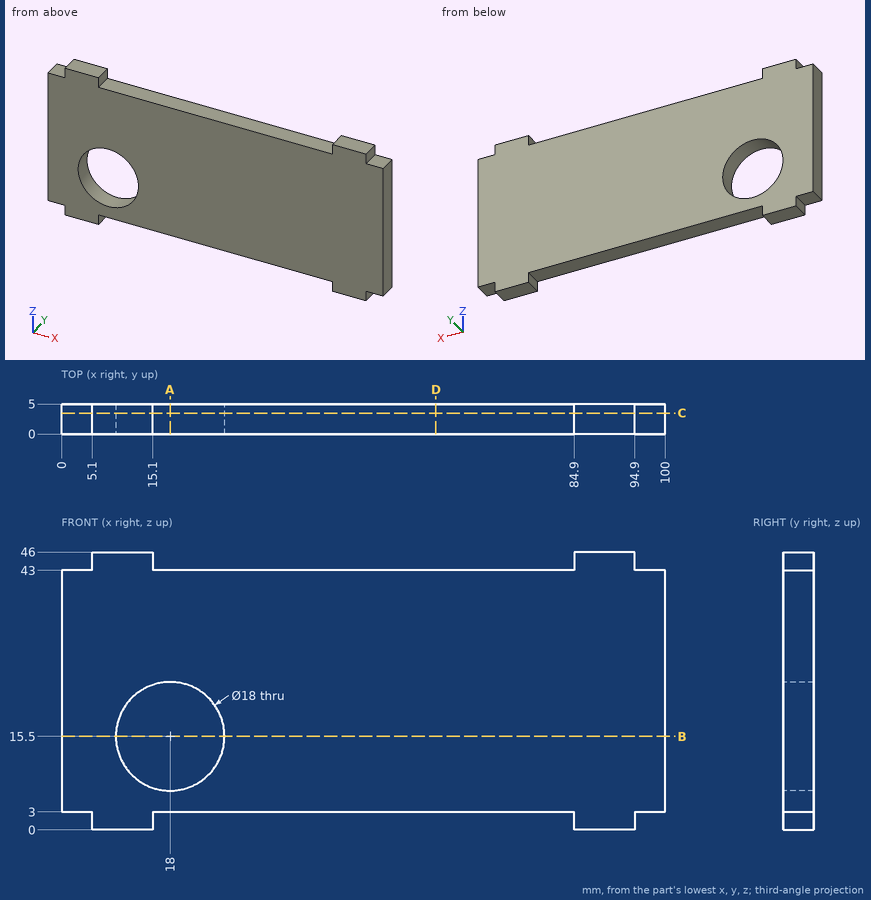
Check sheet for the drawn part. Datum: minimum x, y, z corner. Units: mm. Round coordinates to 2 decimals unless told otherwise and drop trailing zeros. Order: outer loops, then holes, each group sorted by start corner. A loop starts at its lowest first (then second) coordinate and runs counter-clockwise, first axis right, second up.
1) Section check B-B (z = 15.5). Record the boundary of the cut face in (x, y), and give its area (3 significant figures).
2) Go/stop test with flat-tipped pins: pin 1 Ø2.5 at (y, z) = (3, 1.5) entering from -X; pin 2 Ø2.5 at (y, z) = (3, 45) entering from +X; pin 3 Ø1.5 at (x, y) = (38.5, 2) entering from -Z; pin 4 Ø2.5 at (y, z) = (3.5, 2) entering from +X. Record where each tip stops, or that it passes through.
3) Scan lines: line 1 (Z direction, x = 18, y = 2.35); line 2 (X direction, y = 3.8, z = 2); line 3 (Z direction, x = 16.5, y = 3.3). Record each from-to range of solid material in increasing order.
4) Section check A-A (x = 18). Record the boundary of the cut face in (y, z), and give its area (3 significant figures).
5) Section check C-C (y = 3.5). Record the boundary of the cut face in (x, z).
6) Section check D-D (x = 62). Record the boundary of the cut face in (y, z), and give its area (3 significant figures).
Result:
1. outline: (0, 0) - (9, 0) - (9, 5) - (0, 5) - close; (27, 0) - (100, 0) - (100, 5) - (27, 5) - close
1. area: 410 mm2
2. pin 1: stops at x = 5.1
2. pin 2: stops at x = 94.9
2. pin 3: stops at z = 3
2. pin 4: stops at x = 100
3. line 1: z = 3 to 6.5, 24.5 to 43
3. line 2: x = 5.1 to 15.1, 84.9 to 94.9
3. line 3: z = 3 to 6.63, 24.37 to 43
4. outline: (0, 3) - (5, 3) - (5, 6.5) - (0, 6.5) - close; (0, 24.5) - (5, 24.5) - (5, 43) - (0, 43) - close
4. area: 110 mm2
5. outline: (0, 3) - (5.1, 3) - (5.1, 0) - (15.1, 0) - (15.1, 3) - (84.9, 3) - (84.9, 0) - (94.9, 0) - (94.9, 3) - (100, 3) - (100, 43) - (94.9, 43) - (94.9, 46) - (84.9, 46) - (84.9, 43) - (15.1, 43) - (15.1, 46) - (5.1, 46) - (5.1, 43) - (0, 43) - close; hole circle Ø18 at (18, 15.5)
6. outline: (0, 3) - (5, 3) - (5, 43) - (0, 43) - close
6. area: 200 mm2
